```python
from build123d import *

# Parameters (mm, degrees)
F1_DEPTH = 9.525
F2_R     = 2.667
F4_DEPTH = 25.401
F5_W     = 11.93673
F5_H     = 11.176
F6_DEPTH = 15.876


with BuildPart() as f1:
    # F0 (on Top) → F1 (new body, symmetric)
    with BuildSketch(Plane.XY):
        with BuildLine():
            ThreePointArc((-12.824485, 0.254), (0, 12.827), (12.824485, 0.254))
            Line((12.824485, 0.254), (25.39873, 0.254))
            ThreePointArc((25.39873, 0.254), (0, 25.4), (-25.39873, 0.254))
            Line((-25.39873, 0.254), (-12.824485, 0.254))
        make_face()
    extrude(amount=F1_DEPTH, both=True)

    # F2 (on Front) → F4 (cut, through all)
    with BuildSketch(Plane.XZ):
        with Locations((-19.05, 0)):
            Circle(F2_R)
        with Locations((19.05, 0)):
            Circle(F2_R)
    extrude(amount=-F4_DEPTH, mode=Mode.SUBTRACT)

    # F5 (on offset) → F6 (cut, through all)
    with BuildSketch(Plane.XZ.offset(-9.525)):
        with Locations((19.430365, 0)):
            Rectangle(F5_W, F5_H)
        with Locations((-19.430365, 0)):
            Rectangle(F5_W, F5_H)
    extrude(amount=-F6_DEPTH, mode=Mode.SUBTRACT)


solid = f1.part
```
Source: CAD feature listing. Evaluate the final solid. Frame: model axes, mm. A direction names the side the tool comes from. Give positions to 0.01 mm unless a question says otherwise; leave off trailing zeros. Write each loop counter-clockwise with the first axis right and the second up, starting at its lowest first coordinate (ties: lowest second). Pieces come first, ordered by that corner, then holes.
1. First-contact query: pin 1 (1 mm diameter, centred on x = 4.5, z = 2.5, fed in from +Y); pin 2 (8 mm diameter, centred on x = -12, z = 6.5, fed in from +Y); pin 3 (4 mm diameter, centred on x = 9.5, z = -6, fed in from +Y). Flat tips, straight axial feed; report the tip coordinate or a pass-through.
2. Access query for faces 5 (the face through (17, 14, -5.588)), 6 (the face through (-16.506, 4.825, 0.801)), 7 (the face through (-16, 9.525, 0)). Directions: +Z, -Z, +X, -X, +Y, -Y. A direction counts if a zero-diameter tool reaches every point of the face in a straight line with its end or side. Return the directions, or none.
3. Section query B-B (y = 6.25). Return the cut outline in (x, z) (3 decimals).
4. Section query D-D (y = 11.25). Return the cut outline in (x, z) (3 decimals), then the cut area to 3 significant figures.
5. Material intervals for line 1 along Z through (x, y) = (-19.05, 3.75) (3 decimals); line 2 along Z through (x, y) = (18, 11) (3 decimals); line 3 along X through (y, z) = (20.5, 1), sorted ascending.
6. Section query C-C (x = 17). Return the cut outline in (y, z) (3 decimals), then the cut area to 3 significant figures.
7. Pull-direction query (Z, two-part tool) for faces 1 (the face through (0, 13, -9.525)), 2 (the face through (16, 9.525, 0)), 3 (the face through (-22, 0.254, 0)), 4 (the face through (17, 14, 5.588)); classes: +Z half, -Z half, draft (parallel to the pull), parting line (faces both ways), or undercut.
8. Section query A-A (z = 0). Return the cut outline in (x, y) (3 decimals).
Output values:
1. pin 1: stops at y = 25.08
1. pin 2: stops at y = 24.11
1. pin 3: stops at y = 24.27
2. face 5: +X, +Y
2. face 6: +Y, -Y
2. face 7: -X, +Y
3. outline: (-24.619, -9.525) - (-11.201, -9.525) - (-11.201, 9.525) - (-24.619, 9.525) - close; (11.201, -9.525) - (24.619, -9.525) - (24.619, 9.525) - (11.201, 9.525) - close; hole circle Ø5.334 at (-19.05, 0); hole circle Ø5.334 at (19.05, 0)
4. outline: (-22.773, -9.525) - (-6.162, -9.525) - (-6.162, 9.525) - (-22.773, 9.525) - (-22.773, 5.588) - (-13.462, 5.588) - (-13.462, -5.588) - (-22.773, -5.588) - close; (6.162, -9.525) - (22.773, -9.525) - (22.773, -5.588) - (13.462, -5.588) - (13.462, 5.588) - (22.773, 5.588) - (22.773, 9.525) - (6.162, 9.525) - close
4. area: 425 mm2
5. line 1: z = -9.525 to -2.667, 2.667 to 9.525
5. line 2: z = -9.525 to -5.588, 5.588 to 9.525
5. line 3: x = -13.46 to 13.46
6. outline: (0.254, -9.525) - (18.872, -9.525) - (18.872, -5.588) - (9.525, -5.588) - (9.525, -1.706) - (0.254, -1.706) - close; (0.254, 1.706) - (9.525, 1.706) - (9.525, 5.588) - (18.872, 5.588) - (18.872, 9.525) - (0.254, 9.525) - close
6. area: 219 mm2
7. face 1: -Z half
7. face 2: undercut
7. face 3: draft
7. face 4: undercut
8. outline: (-25.399, 0.254) - (-21.717, 0.254) - (-21.717, 9.525) - (-23.546, 9.525) arc R25.4 ccw to start; (-16.383, 0.254) - (-12.824, 0.254) arc R12.827 cw to (12.824, 0.254) - (16.383, 0.254) - (16.383, 9.525) - (13.462, 9.525) - (13.462, 21.539) arc R25.4 ccw to (-13.462, 21.539) - (-13.462, 9.525) - (-16.383, 9.525) - close; (21.717, 0.254) - (25.399, 0.254) arc R25.4 ccw to (23.546, 9.525) - (21.717, 9.525) - close
